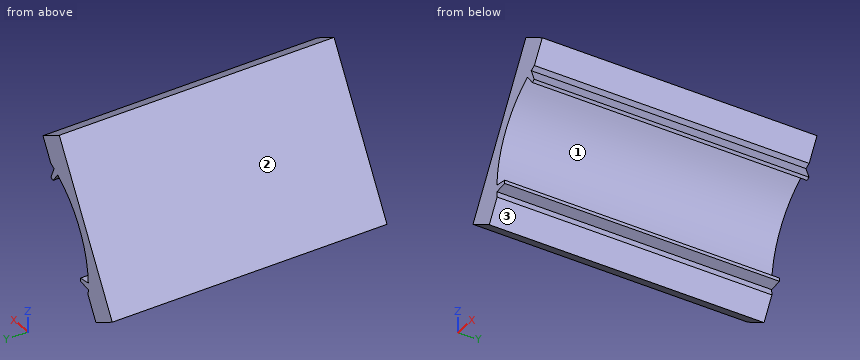
```python
from build123d import *

# Parameters (mm, degrees)
BOSS_EXTRUDE1_DEPTH = 50


with BuildPart() as part:
    # Sketch1 → Boss-Extrude1 (new body)
    with BuildSketch(Plane(origin=(0, 0, 0), x_dir=(1, 0, 0), z_dir=(0, 1, 0))):
        with BuildLine():
            Line((-16.188252967, -0.3), (-16.188252967, 0.3))
            Line((-16.188252967, 0.3), (-18.390214789, 0.6))
            ThreePointArc((-18.390214789, 0.6), (-18.366950287, 1.102332591), (-18.329967032, 1.603841822))
            Line((-18.329967032, 1.603841822), (-20.552991394, 5.454232962))
            Line((-20.552991394, 5.454232962), (-25.166918237, 2.790381057))
            Line((-25.166918237, 2.790381057), (-10.166918237, -23.190381057))
            Line((-10.166918237, -23.190381057), (-5.552991394, -20.526529152))
            Line((-5.552991394, -20.526529152), (-7.776015755, -16.676138011))
            ThreePointArc((-7.776015755, -16.676138011), (-8.228827116, -16.457411834), (-8.675492152, -16.226393189))
            Line((-8.675492152, -16.226393189), (-7.834318863, -14.169438313))
            Line((-7.834318863, -14.169438313), (-8.353934105, -13.869438313))
            Line((-8.353934105, -13.869438313), (-9.714722637, -15.626393189))
            ThreePointArc((-9.714722637, -15.626393189), (-15.93486743, -9.2), (-18.390214789, -0.6))
            Line((-18.390214789, -0.6), (-16.188252967, -0.3))
        make_face()
    extrude(amount=BOSS_EXTRUDE1_DEPTH)


solid = part.part
```
Geometry: final body of the model. Coordinates: model frame, mm. Face numbers are marked on the shaded views. Round coordinates to 2 decimals unless told otherwise and drop trailing zeros. Loops run counter-clockwise (first coordinate to the right, second up) from the corner with the lowest first, then second, coordinate; pieces in that order, holes last.
Item 1: Section A-A, the plane y = 15.5. Output: boundary loops of the cut face in (x, z).
Checked values:
outline: (-25.17, -2.79) - (-20.55, -5.45) - (-18.33, -1.6) arc R18.4 cw to (-18.39, -0.6) - (-16.19, -0.3) - (-16.19, 0.3) - (-18.39, 0.6) arc R18.4 cw to (-9.71, 15.63) - (-8.35, 13.87) - (-7.83, 14.17) - (-8.68, 16.23) arc R18.4 cw to (-7.78, 16.68) - (-5.55, 20.53) - (-10.17, 23.19) - close
Item 2: Contact query for flat-ended pins moving along their axis: P1, Ø1.5, axis at y = 33, z = 11, coming from the +X side; P2, Ø10, axis at x = -16.5, y = 19, coming from the +Z side; P3, Ø3, axis at y = 30, z = 17, coming from the -X side. Output: stop coordinate, or through.
Checked values:
P1: stops at x = -14.16
P2: stops at z = 20.88
P3: stops at x = -14.61
Item 3: Line query: L1, parallel to X at y = 38.5, z = 14; L2, parallel to Z at x = -8.5, y = 43; L3, parallel to X at y = 19, z = 4. Output: solid intervals per line, ascending.
Checked values:
L1: x = -15.47 to -11.94, -8.46 to -8.13
L2: z = 14.06 to 15.8, 16.32 to 22.23
L3: x = -21.25 to -17.96
Item 4: Section B-B, the plane z = 21.5. Output: boundary loops of the cut face in (x, y), plus the area to 3 significant figures.
Checked values:
outline: (-11.14, 0) - (-7.24, 0) - (-7.24, 50) - (-11.14, 50) - close
area: 195 mm2
Item 5: Section C-C, the plane x = -11.5. Output: boundary loops of the cut face in (y, z).
Checked values:
outline: (0, 14.36) - (50, 14.36) - (50, 20.88) - (0, 20.88) - close
Item 6: Mould query, pull axis X, two halves, no side actions, for the marked faces 1, 2 and 3. Classes: released by +X, released by -X, zero draft, split by the parting line, or undercut.
Checked values:
face 1: undercut
face 2: released by -X
face 3: released by +X
